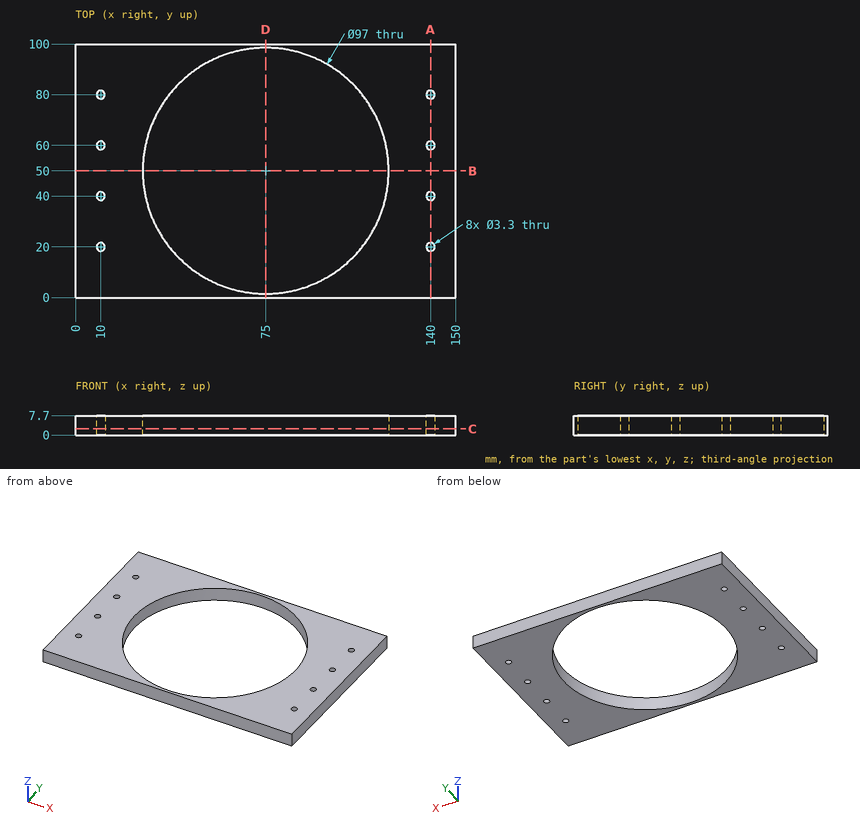
The drawing under review shows one solid part. Ordinate dimensions are in mm from its lowest x, y, z. Give positions to 0.01 mm unless a question says otherwise; leave off trailing zeros. Write each loop counter-clockwise with the first axis right and the second up, starting at its lowest first coordinate (ties: lowest second). Pieces come first, ordered by that corner, then holes. Notation, with made-up numbers: M 10,32 L 54,32 A12 ccw 54,36 Z; hole C 1,9 d2. An arc over 180 degrees is marked long. Write each question's results on one line, items separated by ' | '. Start each with the question number.
1. We need section C-C (z = 2.5). Count the separate pieces of the cut face and the enclosed holes in it, and give its area (3 significant figures).
2. We need section D-D (x = 75). Write out the cut boundary in (y, z), and give its area (3 significant figures).
3. We need section B-B (y = 50). Write out the cut boundary in (x, z).
4. Insertion check: pin 1 Ø3 at (x, y) = (140, 80) entering from -Z. The pin has a flat end and moves straight along its axis. Give the tip position at first contact, or say it passes through.
5. We need section A-A (x = 140). Write out the cut boundary in (y, z), and give its area (3 significant figures).
6. For probe 1 along Y at (x, z) = (140, 3); probe 2 along X at (y, z) = (18, 6); probe 3 along X at (y, z) = (80, 2), list the stretches that pass through material, from the lowest coordinate up. Write a range as [from, to].
Results found:
1) separate pieces: 1 | enclosed holes: 9 | area: 7,540 mm^2
2) outline: M 0,0 L 1.5,0 L 1.5,7.7 L 0,7.7 Z; M 98.5,0 L 100,0 L 100,7.7 L 98.5,7.7 Z | area: 23.1 mm^2
3) outline: M 0,0 L 26.5,0 L 26.5,7.7 L 0,7.7 Z; M 123.5,0 L 150,0 L 150,7.7 L 123.5,7.7 Z
4) pin 1: passes through
5) outline: M 0,0 L 18.35,0 L 18.35,7.7 L 0,7.7 Z; M 21.65,0 L 38.35,0 L 38.35,7.7 L 21.65,7.7 Z; M 41.65,0 L 58.35,0 L 58.35,7.7 L 41.65,7.7 Z; M 61.65,0 L 78.35,0 L 78.35,7.7 L 61.65,7.7 Z; M 81.65,0 L 100,0 L 100,7.7 L 81.65,7.7 Z | area: 668 mm^2
6) probe 1: y = [0, 18.35], [21.65, 38.35], [41.65, 58.35], [61.65, 78.35], [81.65, 100] | probe 2: x = [0, 38.55], [111.45, 150] | probe 3: x = [0, 8.35], [11.65, 36.89], [113.11, 138.35], [141.65, 150]
